```python
from build123d import *

# Parameters (mm, degrees)
EXTRUDE_1_DEPTH = 4
SKETCH_2_W      = 18
SKETCH_2_H      = 65
EXTRUDE_2_DEPTH = 4
FILLET_1_R      = 1


with BuildPart() as part:
    # 草图1 → 凸台-拉伸1 (new body)
    with BuildSketch(Plane(origin=(0, 0, 0), x_dir=(1, 0, 0), z_dir=(0, 1, 0))):
        Polygon((0, -66), (0, 0), (-196, 0), (-196, -82), (-22, -82), (-22, -66), align=None)
    extrude(amount=EXTRUDE_1_DEPTH)

    # 草图2 → 凸台-拉伸2 (add)
    with BuildSketch(Plane(origin=(0, 4, 0), x_dir=(1, 0, 0), z_dir=(0, 1, 0))):
        with Locations((-205, -48.5)):
            Rectangle(SKETCH_2_W, SKETCH_2_H)
    extrude(amount=-EXTRUDE_2_DEPTH)

    # 圆角1
    fillet_1_edges = [part.edges().sort_by_distance(p)[0] for p in [
        (-22, 2, 82),
        (-196, 2, 82),
        (0, 2, 66),
        (-22, 2, 66),
        (-196, 2, 16),
        (-214, 2, 81),
        (-214, 2, 16),
    ]]
    fillet(fillet_1_edges, radius=FILLET_1_R - 0.0001)  # a hair under: the kernel refuses the full size


solid = part.part
```
Read the model definition and answer for the solid it produces. Units are mm, in the model's axes. A direction names the side the tool comes from. Coordinates: 2 decimals unless noted, no trailing zeros. Order: outer loops, then holes, each group sorted by start corner. A loop starts at its lowest first (then second) coordinate and runs counter-clockwise, first axis right, second up. Notation, with made-up numbers: (87, 50.25) - (120, 50.25) arc R22 ccw to (120, 82.25) - close; hole circle Ø8 at (49.5, 35.25). An arc over 180 degrees is marked (long way). Answer as a JSON object with one key per item and string values. Group by question number.
Item 1: Consider probe 1 along X at (y, z) = (2, 67); probe 2 along Z at (x, y) = (-15.5, 1.3). Determine where each line is inside the solid, lowest interval first. Write a range as from..to.
Item 2: Section C-C (x = -14.5) is taken. Give the vertices of the cut face in (y, z).
Item 3: Section B-B (z = 75.5) is taken. Give the vertices of the cut face in (x, y), plus the area to 3 significant figures.
Item 4: A tool of negligible diameter and unlimited length cuts with its end or side. For faces 1 (the face through (-108, 0, 40)), 2 (the face through (-205, 2, 16)), 3 (the face through (-11, 2, 66)), 4 (the face through (-97, 2, 0)), 5 (the face through (-205, 2, 81)), from which of +Z, -Z, +X, -X, +Y, -Y can it reach the whole face along a straight path? Write none if from no direction.
Item 5: Flat-ended cylindrical pins translate along their axes: P1, Ø2, axis at x = -200.5, y = 1, coming from the +Z side; P2, Ø1.2, axis at y = 3, z = 71.5, coming from the +X side; P3, Ø2, axis at x = -206.5, y = 2, coming from the -Z side. Find the tip coordinate at first contact, or state that the pin passes through.
Results are:
{
 "1": {"probe 1": "x = -214..-22", "probe 2": "z = 0..66"},
 "2": {"outline": "(0, 0) - (4, 0) - (4, 66) - (0, 66) - close"},
 "3": {"outline": "(-214, 0) - (-22, 0) - (-22, 4) - (-214, 4) - close", "area": "768 mm^2"},
 "4": {"face 1": "+Z, -Z, +X, -X, -Y", "face 2": "-Z, -X, +Y, -Y", "face 3": "+Z, +X, +Y, -Y", "face 4": "-Z, +X, -X, +Y, -Y", "face 5": "+Z, -X, +Y, -Y"},
 "5": {"P1": "stops at z = 81", "P2": "stops at x = -22", "P3": "stops at z = 16"}
}
